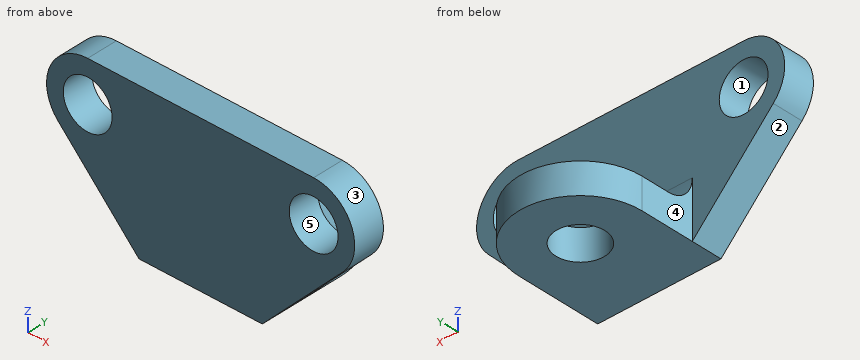
from build123d import *

# Parameters (mm, degrees)
EXTRUDE_3_DEPTH     = 12
SKETCH_10_R         = 9.5
CUT_EXTRUDE_4_DEPTH = 13
EXTRUDE_4_DEPTH     = 12
SKETCH_12_R         = 9.5
CUT_EXTRUDE_5_DEPTH = 12
FILLET_1_R          = 10


with BuildPart() as part:
    # 스케치8 → 보스-돌출3 (new body)
    with BuildSketch(Plane(origin=(0, 0, 0), x_dir=(1, 0, 0), z_dir=(0, 1, 0))):
        with BuildLine():
            Line((-44, -16), (44, -16))
            ThreePointArc((44, -16), (58.715829405, -6.280474897), (55.552799645, 11.069454384))
            Line((55.552799645, 11.069454384), (24, 44))
            Line((24, 44), (-24, 44))
            Line((-24, 44), (-55.552799645, 11.069454384))
            ThreePointArc((-55.552799645, 11.069454384), (-58.715829405, -6.280474897), (-44, -16))
        make_face()
    extrude(amount=EXTRUDE_3_DEPTH)

    # 스케치10 → 컷-돌출4 (cut, through all)
    with BuildSketch(Plane(origin=(0, 0, 0), x_dir=(1, 0, 0), z_dir=(0, 1, 0))):
        with Locations((-44, 0)):
            Circle(SKETCH_10_R)
        with Locations((44, 0)):
            Circle(SKETCH_10_R)
    extrude(amount=CUT_EXTRUDE_4_DEPTH, mode=Mode.SUBTRACT)

    # 스케치11 → 보스-돌출4 (add)
    with BuildSketch(Plane(origin=(0, 0, -44), x_dir=(-1, 0, 0), z_dir=(0, 0, -1))):
        with BuildLine():
            Line((-24, 33), (-24, 0))
            Line((-24, 0), (24, 0))
            Line((24, 0), (24, 33))
            ThreePointArc((24, 33), (0, 57), (-24, 33))
        make_face()
    extrude(amount=-EXTRUDE_4_DEPTH)

    # 스케치12 → 컷-돌출5 (cut)
    with BuildSketch(Plane.XY.offset(-32)):
        with Locations((0, 33)):
            Circle(SKETCH_12_R)
    extrude(amount=-CUT_EXTRUDE_5_DEPTH, mode=Mode.SUBTRACT)

    # 필렛1
    fillet_1_edges = [part.edges().sort_by_distance(p)[0] for p in [
        (0, 12, -32),
    ]]
    fillet(fillet_1_edges, radius=FILLET_1_R)


solid = part.part
Geometry: final body of the model. Coordinates: model frame, mm. Face numbers are marked on the shaded views. A direction names the side the tool comes from. Give positions to 0.01 mm unless a question says otherwise; leave off trailing zeros. Write each loop counter-clockwise with the first axis right and the second up, starting at its lowest first coordinate (ties: lowest second). Pieces come first, ordered by that corner, then holes. Notation, with made-up numbers: (-37, 16.25) -> (5, 16.25) arc R24 cw to (5, 30.25) -> close; hole circle Ø1 at (-36, -23.5). An arc over 180 degrees is marked (long way). Answer in a Markdown table with one row per item.
(1) Draft query along X for the marked faces 1, 2 and 3. Return one class per face: +X half, -X half, draft (parallel to the pull), parting line (faces both ways), or undercut.
Answers below:
| item | result |
|---|---|
| face 1 | undercut |
| face 2 | -X half |
| face 3 | +X half |
(2) Set-up query: the marked faces 4 and 5. Return all of +Z, -Z, +X, -X, +Y, -Y with unobstructed straight access to the full face (end or side cutting, diameter ignored); none if empty.
Answers below:
| item | result |
|---|---|
| face 4 | +Z, -Z, -X, +Y |
| face 5 | +Y, -Y |
(3) Section query D-D on z = -37. Return loops of the section in (x, y).
Answers below:
| item | result |
|---|---|
| outline | (-30.71, 0) -> (30.71, 0) -> (30.71, 12) -> (24, 12) -> (24, 33) arc R24 ccw to (-24, 33) -> (-24, 12) -> (-30.71, 12) -> close; hole circle Ø19 at (0, 33) |
(4) Section query A-A on z = 0. Return loops of the section in (x, y).
Answers below:
| item | result |
|---|---|
| outline | (-60, 0) -> (-53.5, 0) -> (-53.5, 12) -> (-60, 12) -> close; (-34.5, 0) -> (34.5, 0) -> (34.5, 12) -> (-34.5, 12) -> close; (53.5, 0) -> (60, 0) -> (60, 12) -> (53.5, 12) -> close |
(5) Section query B-B on y = 3. Return loops of the section in (x, z).
Answers below:
| item | result |
|---|---|
| outline | (-55.55, -11.07) -> (-24, -44) -> (24, -44) -> (55.55, -11.07) arc R16 ccw to (44, 16) -> (-44, 16) arc R16 ccw to start; hole circle Ø19 at (-44, 0); hole circle Ø19 at (44, 0) |
(6) Section query C-C on x = -7.5. Return loops of the section in (y, z), then the cut area to 3 significant figures.
Answers below:
| item | result |
|---|---|
| outline | (0, -44) -> (27.17, -44) -> (27.17, -32) -> (22, -32) arc R10 cw to (12, -22) -> (12, 16) -> (0, 16) -> close; (38.83, -44) -> (55.8, -44) -> (55.8, -32) -> (38.83, -32) -> close |
| area | 1,130 mm^2 |
(7) Ray query, line 1 along X through (y, z) = (3.5, 0); line 2 along Y through (x, z) = (0, -41); line 3 along Z through (x, y) = (-12, 28.5). Return the intervals inside material, ascending. Write a range as [from, to].
Answers below:
| item | result |
|---|---|
| line 1 | [-60, -53.5], [-34.5, 34.5], [53.5, 60] |
| line 2 | [0, 23.5], [42.5, 57] |
| line 3 | [-44, -32] |
(8) Pin query (flat end, axial travel): pin 1 (15 mm diameter, centred on x = 44, z = 0, fed in from -Y); pin 2 (10 mm diameter, centred on x = -12, y = 22, fed in from +Z); pin 3 (12 mm diameter, centred on x = 13, y = 28, fed in from +Z); pin 4 (23 mm diameter, centred on y = 26.5, z = -27.5, fed in from -X). Return the tip coordinate at first contact, or that it passes through.
Answers below:
| item | result |
|---|---|
| pin 1 | through |
| pin 2 | z = -30.66 |
| pin 3 | z = -32 |
| pin 4 | x = -24 |
